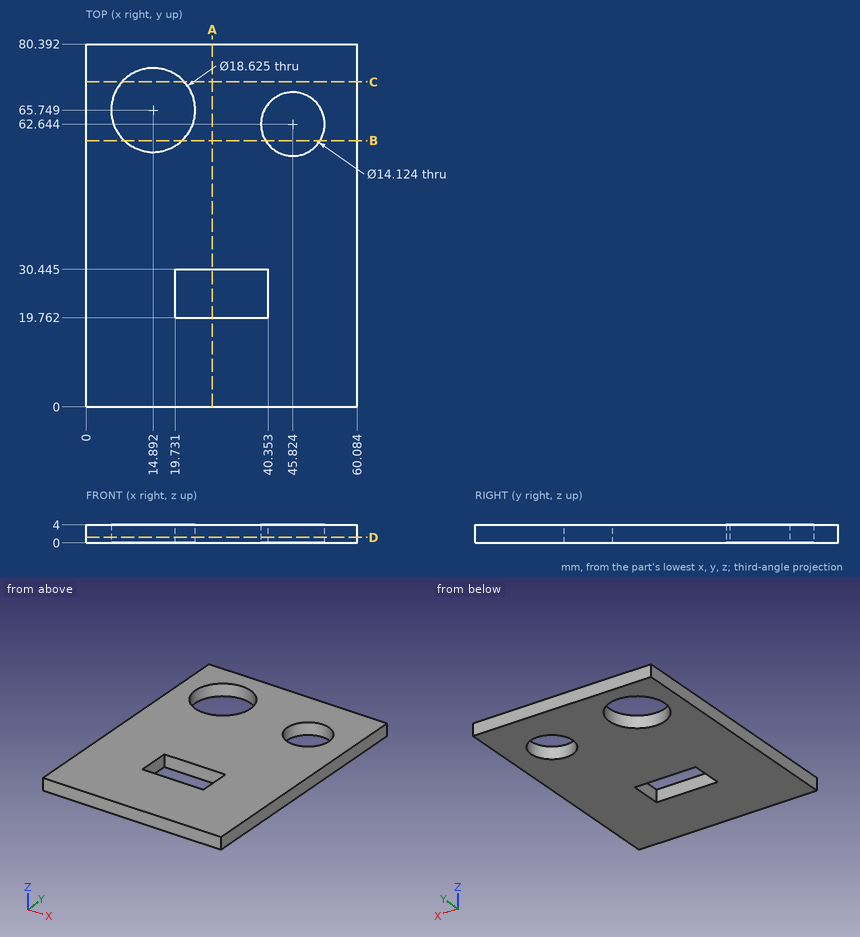
For this review, use the dimensioned drawing (mm, ordinates from the lowest corner) and the shaded views. Coordinates: 2 decimals unless noted, no trailing zeros. Write each loop counter-clockwise with the first axis right and the second up, starting at its lowest first coordinate (ties: lowest second). Pieces come first, ordered by that corner, then holes. Notation, with made-up numbers: (0.25, 58) - (38.25, 58) arc R11 cw to (38.25, 73) - close; hole circle Ø5 at (11.25, 34.5). An arc over 180 degrees is marked (long way). Answer in a Markdown table with one row per item. Add a question column.
Q1. Consider section C-C on y = 72. Give the boundary of the cut face in (x, z) (1 decimal).
Q2. To check wall thickness, follow line 1 along Y through (x, z) = (24.5, 1.15) (1 decimal); line 2 along X through (y, z) = (62.5, 2.2) (1 decimal); line 3 along X through (y, z) = (57.5, 2.85) (1 decimal). State the ranges of each line that lie inside material, in increasing order. Write a range as from..to.
Q3. Consider section D-D on z = 1.2. Give the number of separate pieces and of enclosed holes in the cut face, then the cut area to 3 significant figures.
Q4. Consider section A-A on x = 28. Give the boundary of the cut face in (y, z) (1 decimal).
Q5. Consider section B-B on y = 59. Give the boundary of the cut face in (x, z) (1 decimal), then the cut area to 3 significant figures.
Answers below:
| question | item | result |
|---|---|---|
| 1 | outline | (0, 0) - (8, 0) - (8, 4) - (0, 4) - close; (21.8, 0) - (60.1, 0) - (60.1, 4) - (21.8, 4) - close |
| 2 | line 1 | 0..19.8, 30.4..80.4 |
| 2 | line 2 | 0..6.2, 23.6..38.8, 52.9..60.1 |
| 2 | line 3 | 0..10.6, 19.2..41, 50.7..60.1 |
| 3 | separate pieces | 1 |
| 3 | enclosed holes | 3 |
| 3 | area | 4,180 mm² |
| 4 | outline | (0, 0) - (19.8, 0) - (19.8, 4) - (0, 4) - close; (30.4, 0) - (80.4, 0) - (80.4, 4) - (30.4, 4) - close |
| 5 | outline | (0, 0) - (8.5, 0) - (8.5, 4) - (0, 4) - close; (21.3, 0) - (39.8, 0) - (39.8, 4) - (21.3, 4) - close; (51.9, 0) - (60.1, 0) - (60.1, 4) - (51.9, 4) - close |
| 5 | area | 141 mm² |
